from build123d import *
from build123d.topology import SkipClean

# Parameters (mm, degrees)
SKETCH1_R           = 36.85
BOSS_EXTRUDE1_DEPTH = 15
SKETCH2_R           = 2.25
CUT_EXTRUDE1_DEPTH  = 87.187940965
BOSS_EXTRUDE2_DEPTH = 20
FILLET1_R           = 10
CUT_EXTRUDE2_START  = -6
CUT_EXTRUDE2_DEPTH  = 6
SKETCH5_R           = 1.75
CUT_EXTRUDE3_DEPTH  = 92.806106375
FILLET2_R           = 10


with BuildPart() as part:
    # Sketch1 → Boss-Extrude1 (new body)
    with BuildSketch(Plane(origin=(0, 0, 0), x_dir=(1, 0, 0), z_dir=(0, 1, 0))):
        with BuildLine():
            Line((-70.770323355, -10), (-45.770323355, -10))
            ThreePointArc((-45.770323355, -10), (46.85, 0), (-45.770323355, 10))
            Line((-45.770323355, 10), (-70.770323355, 10))
            Line((-70.770323355, 10), (-70.770323355, -10))
        make_face()
        with Locations(Location((0, 0, 0), (0, 0, 270))):
            Circle(SKETCH1_R, mode=Mode.SUBTRACT)
    extrude(amount=BOSS_EXTRUDE1_DEPTH)

    # Sketch2 → Cut-Extrude1 (cut, through all)
    with BuildSketch(Plane(origin=(0, 15, 0), x_dir=(1, 0, 0), z_dir=(0, 1, 0))):
        with Locations(Location((-63.770323355, 0, 0), (0, 0, 270))):
            Circle(SKETCH2_R)
        with Locations(Location((-48.770323355, 0, 0), (0, 0, 270))):
            Circle(SKETCH2_R)
    extrude(amount=-CUT_EXTRUDE1_DEPTH, mode=Mode.SUBTRACT)

    # Sketch3 → Boss-Extrude2 (add)
    with SkipClean():  # the faces are left unmerged after this step: merging them gives an invalid solid
        with BuildSketch(Plane(origin=(0, 15, 0), x_dir=(1, 0, 0), z_dir=(0, 1, 0))):
            with BuildLine():
                ThreePointArc((-1.85, -36.803532439), (-3.352802058, -36.697155453), (-4.85, -36.529440182))
                Line((-4.85, -36.529440182), (-4.85, -46.59828323))
                ThreePointArc((-4.85, -46.59828323), (-3.351727199, -46.729952116), (-1.85, -46.813459603))
                Line((-1.85, -46.813459603), (-1.85, -36.803532439))
            make_face()
            with BuildLine():
                ThreePointArc((1.85, -46.813459603), (3.351727199, -46.729952116), (4.85, -46.59828323))
                Line((4.85, -46.59828323), (4.85, -36.529440182))
                ThreePointArc((4.85, -36.529440182), (3.352802058, -36.697155453), (1.85, -36.803532439))
                Line((1.85, -36.803532439), (1.85, -46.813459603))
            make_face()
            with BuildLine():
                ThreePointArc((4.85, 46.59828323), (3.351727199, 46.729952116), (1.85, 46.813459603))
                Line((1.85, 46.813459603), (1.85, 36.803532439))
                ThreePointArc((1.85, 36.803532439), (3.352802058, 36.697155453), (4.85, 36.529440182))
                Line((4.85, 36.529440182), (4.85, 46.59828323))
            make_face()
            with BuildLine():
                Line((-1.85, 36.803532439), (-1.85, 46.813459603))
                ThreePointArc((-1.85, 46.813459603), (-3.351727199, 46.729952116), (-4.85, 46.59828323))
                Line((-4.85, 46.59828323), (-4.85, 36.529440182))
                ThreePointArc((-4.85, 36.529440182), (-3.352802058, 36.697155453), (-1.85, 36.803532439))
            make_face()
        extrude(amount=BOSS_EXTRUDE2_DEPTH)

    # Fillet1
    # the kernel refuses this fillet: 10 mm, written as the material it adds along each edge
    with BuildSketch(Plane(origin=(-4.85, 15, 11.529440182), x_dir=(-1, 0, 0), z_dir=(0, 0, 1))) as fillet1_piece_1_section:
        with BuildLine():
            CenterArc((FILLET1_R, -FILLET1_R), FILLET1_R, 90, 90)
            Line((0, -FILLET1_R), (0, 0))
            Line((0, 0), (FILLET1_R, 0))
        make_face()
    fillet1_piece_1 = extrude(amount=60.068843048, mode=Mode.PRIVATE)
    fillet1_piece_1 = fillet1_piece_1 & Plane(origin=(0, 17.250913244, 0), x_dir=(-0.9769546073589704, 0, 0.2134471718249741), z_dir=(0, -1, 0)) * Cylinder(46.85, 161, mode=Mode.PRIVATE)
    fillet1_piece_1 = fillet1_piece_1 - Plane(origin=(0, 17.250913244, 0), x_dir=(0, 0, 1), z_dir=(0, -1, 0)) * Cylinder(36.85, 161, mode=Mode.PRIVATE)
    with BuildSketch(Plane(origin=(4.85, 15, 71.59828323), x_dir=(1, 0, 0), z_dir=(0, 0, -1))) as fillet1_piece_2_section:
        with BuildLine():
            CenterArc((FILLET1_R, -FILLET1_R), FILLET1_R, 90, 90)
            Line((0, -FILLET1_R), (0, 0))
            Line((0, 0), (FILLET1_R, 0))
        make_face()
    fillet1_piece_2 = extrude(amount=60.068843048, mode=Mode.PRIVATE)
    fillet1_piece_2 = fillet1_piece_2 & Plane(origin=(0, 17.250905791, 0), x_dir=(-0.9769546073589704, 0, 0.2134471718249741), z_dir=(0, -1, 0)) * Cylinder(46.85, 161, mode=Mode.PRIVATE)
    fillet1_piece_2 = fillet1_piece_2 - Plane(origin=(0, 17.250905791, 0), x_dir=(0, 0, 1), z_dir=(0, -1, 0)) * Cylinder(36.85, 161, mode=Mode.PRIVATE)
    with BuildSketch(Plane(origin=(4.85, 15, -11.529440182), x_dir=(1, 0, 0), z_dir=(0, 0, -1))) as fillet1_piece_3_section:
        with BuildLine():
            CenterArc((FILLET1_R, -FILLET1_R), FILLET1_R, 90, 90)
            Line((0, -FILLET1_R), (0, 0))
            Line((0, 0), (FILLET1_R, 0))
        make_face()
    fillet1_piece_3 = extrude(amount=60.068843048, mode=Mode.PRIVATE)
    fillet1_piece_3 = fillet1_piece_3 & Plane(origin=(0, 17.250913244, 0), x_dir=(-0.9769546073589704, 0, 0.2134471718249741), z_dir=(0, -1, 0)) * Cylinder(46.85, 161, mode=Mode.PRIVATE)
    fillet1_piece_3 = fillet1_piece_3 - Plane(origin=(0, 17.250913244, 0), x_dir=(0, 0, 1), z_dir=(0, -1, 0)) * Cylinder(36.85, 161, mode=Mode.PRIVATE)
    with BuildSketch(Plane(origin=(-4.85, 15, -71.59828323), x_dir=(-1, 0, 0), z_dir=(0, 0, 1))) as fillet1_piece_4_section:
        with BuildLine():
            CenterArc((FILLET1_R, -FILLET1_R), FILLET1_R, 90, 90)
            Line((0, -FILLET1_R), (0, 0))
            Line((0, 0), (FILLET1_R, 0))
        make_face()
    fillet1_piece_4 = extrude(amount=60.068843048, mode=Mode.PRIVATE)
    fillet1_piece_4 = fillet1_piece_4 & Plane(origin=(0, 17.250905791, 0), x_dir=(-0.9769546073589704, 0, 0.2134471718249741), z_dir=(0, -1, 0)) * Cylinder(46.85, 161, mode=Mode.PRIVATE)
    fillet1_piece_4 = fillet1_piece_4 - Plane(origin=(0, 17.250905791, 0), x_dir=(0, 0, 1), z_dir=(0, -1, 0)) * Cylinder(36.85, 161, mode=Mode.PRIVATE)
    add([fillet1_piece_1, fillet1_piece_2, fillet1_piece_3, fillet1_piece_4])

    # Sketch4 → Cut-Extrude2 (cut)
    with BuildSketch(Plane(origin=(0, 15, 0), x_dir=(1, 0, 0), z_dir=(0, 1, 0)).offset(CUT_EXTRUDE2_START)):
        with BuildLine():
            Line((-1.85, 46.813459603), (-1.85, 36.803532439))
            ThreePointArc((-1.85, 36.803532439), (0, 36.85), (1.85, 36.803532439))
            Line((1.85, 36.803532439), (1.85, 46.813459603))
            ThreePointArc((1.85, 46.813459603), (0, 46.85), (-1.85, 46.813459603))
        make_face()
        with BuildLine():
            Line((1.85, -46.813459603), (1.85, -36.803532439))
            ThreePointArc((1.85, -36.803532439), (0, -36.85), (-1.85, -36.803532439))
            Line((-1.85, -36.803532439), (-1.85, -46.813459603))
            ThreePointArc((-1.85, -46.813459603), (0, -46.85), (1.85, -46.813459603))
        make_face()
    extrude(amount=CUT_EXTRUDE2_DEPTH, mode=Mode.SUBTRACT)

    # Sketch5 → Cut-Extrude3 (cut, symmetric)
    with BuildSketch(Plane(origin=(0, 0, 0), x_dir=(0, 0, -1), z_dir=(1, 0, 0))):
        with Locations(Location((-41.6, 28, 0), (0, 0, 180))):
            Circle(SKETCH5_R)
    cut_extrude3 = extrude(amount=CUT_EXTRUDE3_DEPTH, both=True, mode=Mode.SUBTRACT)

    # Fillet2
    fillet2_edges = [part.edges().sort_by_distance(p)[0] for p in [
        (-45.770323355, 7.5, 10),
        (-45.770323355, 7.5, -10),
    ]]
    fillet(fillet2_edges, radius=FILLET2_R)

    # Mirror1: Cut-Extrude3 across plane
    add(cut_extrude3.mirror(Plane.XY), mode=Mode.SUBTRACT)


solid = part.part
Model file for the job. Use its own axes, mm. A direction names the side the tool comes from. Round coordinates to 2 decimals unless told otherwise and drop trailing zeros. Loops run counter-clockwise (first coordinate to the right, second up) from the corner with the lowest first, then second, coordinate; pieces in that order, holes last.
1. Band-saw the part on B-B, the plane z = 0. List the corners of the cut face in (x, y).
Check values:
outline: (-70.77, 0) - (-66.02, 0) - (-66.02, 15) - (-70.77, 15) - close; (-61.52, 0) - (-51.02, 0) - (-51.02, 15) - (-61.52, 15) - close; (-46.52, 0) - (-36.85, 0) - (-36.85, 15) - (-46.52, 15) - close; (36.85, 0) - (46.85, 0) - (46.85, 15) - (36.85, 15) - close
2. Band-saw the part on A-A, the plane y = 11. List the corners of the cut face in (x, z).
Check values:
outline: (-70.77, -10) - (-53.22, -10) arc R10 cw to (-43.86, -16.48) arc R46.85 ccw to (-1.85, -46.81) - (-1.85, -36.8) arc R36.85 cw to (-1.85, 36.8) - (-1.85, 46.81) arc R46.85 ccw to (-43.86, 16.48) arc R10 cw to (-53.22, 10) - (-70.77, 10) - close; (1.85, -46.81) arc R46.85 ccw to (1.85, 46.81) - (1.85, 36.8) arc R36.85 cw to (1.85, -36.8) - close; hole circle Ø4.5 at (-63.77, 0); hole circle Ø4.5 at (-48.77, 0)
3. Tool access for faces 1 (the flat face through (-62, 7, 10)), 2 (the flat face through (0, 9, -42)), 3 (the flat face through (-4.85, 30, 41)), 4 (the flat face through (4.85, 30, 42)): list every direction of +Z, -Z, +X, -X, +Y, -Y with a clear straight run to the whole face (end or side of a thin tool).
Check values:
face 1: +Z, -X, +Y, -Y
face 2: +Z, -Z, +Y
face 3: +Z, -Z, -X, +Y
face 4: +Z, -Z, +X, +Y
4. Band-saw the part on C-C, the plane x = -18. List the corners of the cut face in (y, z), and give its area (3 significant figures).
Check values:
outline: (0, -43.25) - (15, -43.25) - (15, -32.15) - (0, -32.15) - close; (0, 32.15) - (15, 32.15) - (15, 43.25) - (0, 43.25) - close
area: 333 mm2
5. Drop flat-ended pins along their axis: P1, Ø3, axis at y = 28, z = 41.6, coming from the -X side; P2, Ø12, axis at x = -60, y = 10, coming from the +Z side; P3, Ø11, axis at y = 26, z = -42.5, coming from the -X side; P4, Ø8, axis at y = 29.5, z = -42, coming from the -X side. Give the stop position or say it passes through.
Check values:
P1: passes through
P2: stops at z = 10
P3: stops at x = -5.92
P4: stops at x = -4.85
6. Mould opens along Y. For faces 5 (the cylindrical face through (7.86, 17.85, 40.25)), 6 (the cylindrical face through (-46.54, 7.6, -0.29)), 7 (the cylindrical face through (3.371, 27.474, -43.269)) say: +Y half, -Y half, draft (parallel to the pull), parting line (faces both ways), or undercut.
Check values:
face 5: +Y half
face 6: draft
face 7: undercut
7. Wall check: probe 1 along X at (y, z) = (8.5, 0); probe 2 along Z at (x, y) = (-2, 23.5); probe 3 along X at (y, z) = (31, 41). Give the ranges that are in metal, low to high.
Check values:
probe 1: x = -70.77 to -66.02, -61.52 to -51.02, -46.52 to -36.85, 36.85 to 46.85
probe 2: z = -46.81 to -36.8, 36.8 to 46.81
probe 3: x = -4.85 to -1.85, 1.85 to 4.85
8. Band-saw the part on D-D, the plane y = 28. Count the separate pieces of the cut face and the enclosed holes in it, and give its area (3 significant figures).
Check values:
separate pieces: 8
enclosed holes: 0
area: 78.4 mm2
